from build123d import *

# Parameters (mm, degrees)
SKETCH1_W           = 234.95
SKETCH1_H           = 6.35
BOSS_EXTRUDE1_DEPTH = 256.54
CUT_EXTRUDE1_REACH  = 284.229
SKETCH2_R           = 11.1125


with BuildPart() as part:
    # Sketch1 → Boss-Extrude1 (new body)
    with BuildSketch(Plane.XY):
        Rectangle(SKETCH1_W, SKETCH1_H)
    extrude(amount=BOSS_EXTRUDE1_DEPTH)

    # Sketch2 → Cut-Extrude1 (cut, up to next)
    with BuildSketch(Plane.XZ.offset(3.175), mode=Mode.PRIVATE) as cut_extrude1_sk1:
        with Locations((-63.754, 191.77)):
            Circle(SKETCH2_R)
    cut_extrude1_tool1 = extrude(cut_extrude1_sk1.sketch, amount=-CUT_EXTRUDE1_REACH, mode=Mode.PRIVATE) & part.part
    # Sketch2 → Cut-Extrude1 (cut, up to next)
    with BuildSketch(Plane.XZ.offset(3.175), mode=Mode.PRIVATE) as cut_extrude1_sk2:
        with Locations((-63.754, 64.77)):
            Circle(SKETCH2_R)
    cut_extrude1_tool2 = extrude(cut_extrude1_sk2.sketch, amount=-CUT_EXTRUDE1_REACH, mode=Mode.PRIVATE) & part.part
    # Sketch2 → Cut-Extrude1 (cut, up to next)
    with BuildSketch(Plane.XZ.offset(3.175), mode=Mode.PRIVATE) as cut_extrude1_sk3:
        with Locations((63.754, 64.77)):
            Circle(SKETCH2_R)
    cut_extrude1_tool3 = extrude(cut_extrude1_sk3.sketch, amount=-CUT_EXTRUDE1_REACH, mode=Mode.PRIVATE) & part.part
    # Sketch2 → Cut-Extrude1 (cut, up to next)
    with BuildSketch(Plane.XZ.offset(3.175), mode=Mode.PRIVATE) as cut_extrude1_sk4:
        with Locations((63.754, 191.77)):
            Circle(SKETCH2_R)
    cut_extrude1_tool4 = extrude(cut_extrude1_sk4.sketch, amount=-CUT_EXTRUDE1_REACH, mode=Mode.PRIVATE) & part.part
    add(cut_extrude1_tool1.solids().sort_by_distance((-63.754, -3.175, 191.77))[0], mode=Mode.SUBTRACT)
    add(cut_extrude1_tool2.solids().sort_by_distance((-63.754, -3.175, 64.77))[0], mode=Mode.SUBTRACT)
    add(cut_extrude1_tool3.solids().sort_by_distance((63.754, -3.175, 64.77))[0], mode=Mode.SUBTRACT)
    add(cut_extrude1_tool4.solids().sort_by_distance((63.754, -3.175, 191.77))[0], mode=Mode.SUBTRACT)


solid = part.part
Input: part model. Units: mm. Frame: model coordinates. Give positions to 0.01 mm unless a question says otherwise; leave off trailing zeros. Loops run counter-clockwise (first coordinate to the right, second up) from the corner with the lowest first, then second, coordinate; pieces in that order, holes last. Notation, with made-up numbers: M 59,47 L 89,47 A7 ccw 89,56 Z; hole C -1.5,58.5 d1. An arc over 180 degrees is marked long. Use CSV: the item, a comma, the result in double quotes.
(1) Pull-direction query (X, two-part tool) for faces 1 (the face through (-117.475, 0, 126)), 2 (the face through (117.475, 0, 126)), 3 (the face through (-2, 0, 256.54)), 4 (the face through (-72.572, -0.044, 58.008)); classes: pulls with the +X half, pulls with the -X half, needs draft (parallel to the pull), parting line crosses it, or undercut.
Outcome:
face 1,"pulls with the -X half"
face 2,"pulls with the +X half"
face 3,"needs draft"
face 4,"undercut"
(2) Material intervals for L1, parallel to Z at x = 72, y = -0.25; L2, parallel to Z at x = -68, y = -0.75, sorted ascending. Write a range as [from, to].
Outcome:
L1,"z = [0, 57.32], [72.22, 184.32], [199.22, 256.54]"
L2,"z = [0, 54.5], [75.04, 181.5], [202.04, 256.54]"
(3) Section B-B, the plane y = 2. Return loops of the section in (x, z) (1 decimal).
Outcome:
outline,"M -117.5,0 L 117.5,0 L 117.5,256.5 L -117.5,256.5 Z; hole C -63.8,64.8 d22.2; hole C -63.8,191.8 d22.2; hole C 63.8,64.8 d22.2; hole C 63.8,191.8 d22.2"
(4) Section A-A, the plane z = 191.77. Return loops of the section in (x, y) (1 decimal).
Outcome:
outline,"M -117.5,-3.2 L -74.9,-3.2 L -74.9,3.2 L -117.5,3.2 Z; M -52.6,-3.2 L 52.6,-3.2 L 52.6,3.2 L -52.6,3.2 Z; M 74.9,-3.2 L 117.5,-3.2 L 117.5,3.2 L 74.9,3.2 Z"
(5) Pin query (flat end, axial travel): P1, Ø20, axis at x = -63.754, z = 191.77, coming from the +Y side; P2, Ø1.5, axis at x = -90.5, y = 0, coming from the -Z side. Return the tip coordinate at first contact, or that it passes through.
Outcome:
P1,"passes through"
P2,"stops at z = 0"
